Part print with two shaded views. Sizes in mm from the minimum x, y, z corner. Give positions to 0.01 mm unless a question says otherwise; leave off trailing zeros. Order: outer loops, then holes, each group sorted by start corner. A loop starts at its lowest first (then second) coordinate and runs counter-clockwise, first axis right, second up. Notation, with made-up numbers: M 11,73.25 L 47,73.25 A14 ccw 47,95.25 Z; hole C 49,35 d9. An arc over 180 degrees is marked long. Return JSON: item names as keys, results as strings. Group by question number.
1. Slice it at B-B on z = 1.27. List the corners of the cut face in (x, y), then the cut area to 3 significant figures.
2. Slice it at D-D on x = 1.27. List the corners of the cut face in (y, z), then the cut area to 3 significant figures.
3. Pin check, flat tips, straight feed: pin 1 (2 mm diameter, centred on x = 2.5, y = 3, fed in from +Z); pin 2 (6 mm diameter, centred on x = 15, z = 4.5, fed in from +Y); pin 3 (0.8 mm diameter, centred on y = 2.5, z = 10.5, fed in from +X). Stop position of each tip, or through.
4. Slice it at C-C on z = 6.25. List the corners of the cut face in (x, y).
5. Slice it at A-A on x = 41.91. List the corners of the cut face in (y, z).
6. Wall check: probe 1 along X at (y, z) = (1.2, 1.27); probe 2 along Y at (x, z) = (2.5, 16.75); probe 3 along X at (y, z) = (3.9, 10.75). Give the ranges that are in metal, low to high. Write a range as [from, to].
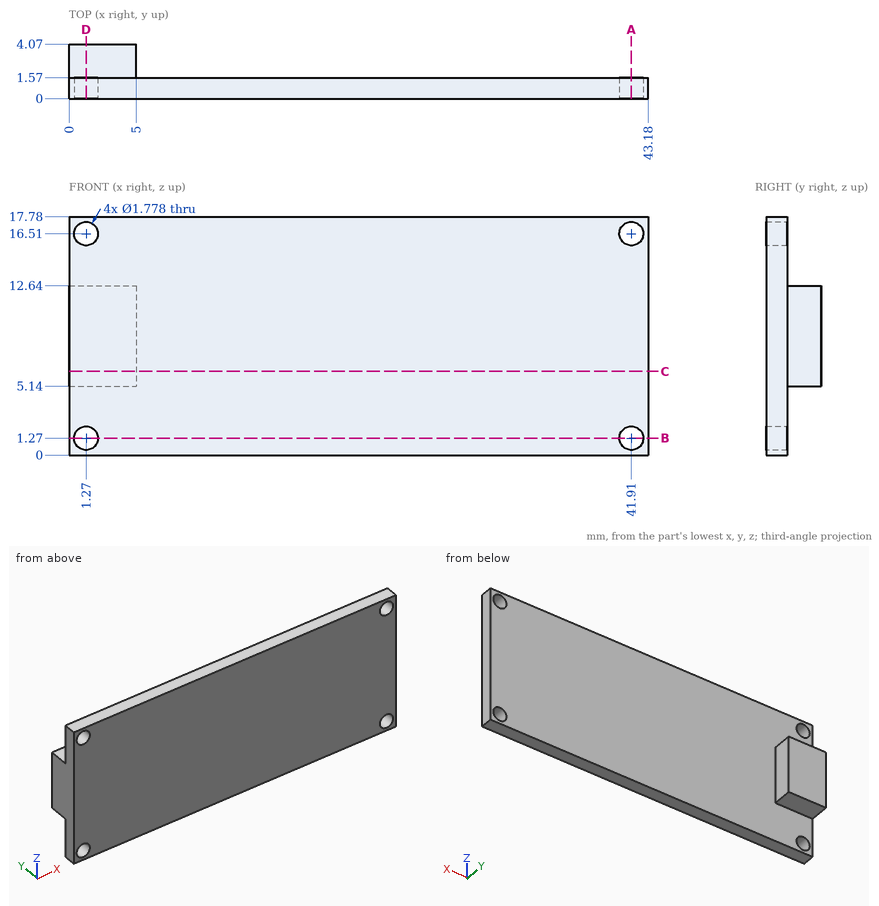
Result:
{
 "1": {"outline": "M 0,0 L 0.38,0 L 0.38,1.57 L 0,1.57 Z; M 2.16,0 L 41.02,0 L 41.02,1.57 L 2.16,1.57 Z; M 42.8,0 L 43.18,0 L 43.18,1.57 L 42.8,1.57 Z", "area": "62.2 mm2"},
 "2": {"outline": "M 0,0 L 1.57,0 L 1.57,0.38 L 0,0.38 Z; M 0,2.16 L 1.57,2.16 L 1.57,5.14 L 4.07,5.14 L 4.07,12.64 L 1.57,12.64 L 1.57,15.62 L 0,15.62 Z; M 0,17.4 L 1.57,17.4 L 1.57,17.78 L 0,17.78 Z", "area": "41.1 mm2"},
 "3": {"pin 1": "stops at z = 12.64", "pin 2": "stops at y = 1.57", "pin 3": "stops at x = 5"},
 "4": {"outline": "M 0,0 L 43.18,0 L 43.18,1.57 L 5,1.57 L 5,4.07 L 0,4.07 Z"},
 "5": {"outline": "M 0,0 L 1.57,0 L 1.57,0.38 L 0,0.38 Z; M 0,2.16 L 1.57,2.16 L 1.57,15.62 L 0,15.62 Z; M 0,17.4 L 1.57,17.4 L 1.57,17.78 L 0,17.78 Z"},
 "6": {"probe 1": "x = [0, 0.38], [2.16, 41.02], [42.8, 43.18]", "probe 2": "y = [0, 1.57]", "probe 3": "x = [0, 5]"}
}
